Geometry check sheet. Reference: the model listing, model coordinates, mm. A direction names the side the tool comes from. Give positions to 0.01 mm unless a question says otherwise; leave off trailing zeros. Write each loop counter-clockwise with the first axis right and the second up, starting at its lowest first coordinate (ties: lowest second). Pieces come first, ordered by that corner, then holes. Notation, with made-up numbers: M 33,-9.5 L 64,-9.5 A10 cw 64,4.5 Z; hole C -6,-11 d8. An arc over 180 degrees is marked long. One line per item, written item: value. Start each with the question number.
1. Release check for a two-part mould opening along X. For faces 1 (the face through (4.62, 5.71, -1.97)), 2 (the face through (-6.2, 3, -2)), 3 (the face through (17, 3, -10)) record: pulls with the +X half, pulls with the -X half, needs draft (parallel to the pull), parting line crosses it, or undercut.
2. Cross-section at A-A on y = 4. Record the cut outline in (x, z).
3. Tool access check on faces 4 (the face through (4.5, 6.2, -3.6)), 5 (the face through (33.8, 3, -5)), 6 (the face through (7, 6, -4.497)), 7 (the face through (-3, 3, -7)). Record the directions out of +Z, -Z, +X, -X, +Y, -Y that give a thin tool (end or side, any length) a straight path to the whole face; none if there is none.
4. Cross-section at B-B on z = -5. Record the cut outline in (x, y), then the cut area to 3 significant figures.
5. Gauge pin test, flat ends, axial feed: pin 1 (3 mm diameter, centred on x = 37, y = 4.5, fed in from +Z); pin 2 (1 mm diameter, centred on y = 5, z = -4, fed in from +X). Record the tip position at first contact, or that the pin passes through.
6. Scan lines: line 1 (Z direction, x = 34.5, y = 1.75); line 2 (X direction, y = 2.5, z = -6.25). Record each from-to range of solid material in increasing order.
from build123d import *

# Parameters (mm, degrees)
BOSS_EXTRUDE1_DEPTH = 6.2
CUT_EXTRUDE1_DEPTH  = 1


with BuildPart() as part:
    # Sketch1 → Boss-Extrude1 (new body)
    with BuildSketch(Plane(origin=(0, 0, 0), x_dir=(1, 0, 0), z_dir=(0, 1, 0))):
        Polygon((0, 0), (33.7, 0), (39.9, 0), (39.9, 3), (33.8, 3), (33.8, 7), (39.9, 7), (39.9, 10), (33.7, 10), (0, 10), (-6.2, 10), (-6.2, 7), (0.1, 7), (0.1, 3), (-6.2, 3), (-6.2, 0), align=None)
    extrude(amount=BOSS_EXTRUDE1_DEPTH)

    # Sketch2 → Cut-Extrude1 (cut)
    with BuildSketch(Plane(origin=(0, 6.2, 0), x_dir=(1, 0, 0), z_dir=(0, 1, 0))):
        with BuildLine():
            Line((4.122268508, 1.240803577), (3.894574197, 1.399171966))
            Line((3.894574197, 1.399171966), (4.777366665, 2.689651734))
            add(Edge.make_bspline(
                [(4.777366665, 2.689651734), (4.721041498, 2.682763741), (4.610134103, 2.669200898), (4.498431161, 2.66670929), (4.443457411, 2.665483064)],
                knots=[0, 0, 0, 0, 0.000170115, 0.000334967, 0.000334967, 0.000334967, 0.000334967], degree=3))
            add(Edge.make_bspline(
                [(4.443457411, 2.665483064), (4.410127124, 2.666336755), (4.344702687, 2.668012475), (4.248516831, 2.681294687), (4.156092072, 2.701750875), (4.067673442, 2.732275102), (3.982928606, 2.770210192), (3.902042566, 2.817251911), (3.825124208, 2.872593333), (3.752999629, 2.935941833), (3.687402552, 3.00549978), (3.628961417, 3.079119542), (3.580391962, 3.157656315), (3.540045345, 3.239508014), (3.509447005, 3.325851097), (3.487165275, 3.415703053), (3.473447139, 3.509693614), (3.471815102, 3.573669982), (3.470986457, 3.606153136)],
                knots=[0, 0, 0, 0, 9.9954e-05, 0.000196201, 0.000290782, 0.000383503, 0.000476303, 0.000568919, 0.000663705, 0.000760153, 0.000856434, 0.000950205, 0.001041624, 0.001132931, 0.001223461, 0.001315861, 0.001410305, 0.001507717, 0.001507717, 0.001507717, 0.001507717], degree=3))
            add(Edge.make_bspline(
                [(3.470986457, 3.606153136), (3.472559837, 3.6505747), (3.475648063, 3.737765218), (3.500502432, 3.865158708), (3.541378597, 3.985615073), (3.598372911, 4.098817606), (3.670159408, 4.203137891), (3.756436486, 4.2971257), (3.856679368, 4.379444246), (3.968604485, 4.450205088), (4.089574726, 4.507114693), (4.216274151, 4.549060344), (4.34773196, 4.573733494), (4.436784061, 4.576986382), (4.481618468, 4.57862409)],
                knots=[0, 0, 0, 0, 0.000133185, 0.000261414, 0.000387724, 0.00051373, 0.000640399, 0.00076644, 0.000895188, 0.001028407, 0.001162697, 0.001295241, 0.001427846, 0.0015623, 0.0015623, 0.0015623, 0.0015623], degree=3))
            add(Edge.make_bspline(
                [(4.481618468, 4.57862409), (4.525604392, 4.57696387), (4.612516431, 4.573683434), (4.740322887, 4.54965869), (4.862733666, 4.509166851), (4.97907019, 4.45321014), (5.0867838, 4.383069031), (5.183644714, 4.299489856), (5.267442525, 4.202420556), (5.338039902, 4.094208854), (5.394709153, 3.977943093), (5.435596152, 3.856581963), (5.460765411, 3.730998266), (5.463937079, 3.645913279), (5.465537739, 3.602973048)],
                knots=[0, 0, 0, 0, 0.000131915, 0.000260652, 0.000388569, 0.000517718, 0.000646848, 0.000773094, 0.000900237, 0.001030248, 0.001159674, 0.001287189, 0.001413545, 0.001542287, 0.001542287, 0.001542287, 0.001542287], degree=3))
            add(Edge.make_bspline(
                [(5.465537739, 3.602973048), (5.464468754, 3.569641202), (5.462300585, 3.50203589), (5.447118363, 3.399319794), (5.421337195, 3.294589035), (5.392080297, 3.205941588), (5.363838974, 3.132727494), (5.337258661, 3.074895704), (5.307765493, 3.014025272), (5.273367756, 2.950754473), (5.23639053, 2.884276745), (5.194608186, 2.815258852), (5.148973846, 2.74360818), (5.116471172, 2.695305464), (5.099827603, 2.670571205)],
                knots=[0, 0, 0, 0, 9.9984e-05, 0.000202793, 0.000310776, 0.000423207, 0.000482616, 0.000546097, 0.000614079, 0.0006855, 0.000762103, 0.000842274, 0.000927493, 0.001016928, 0.001016928, 0.001016928, 0.001016928], degree=3))
            Line((5.099827603, 2.670571205), (4.122268508, 1.240803577))
        make_face()
        with BuildLine():
            add(Edge.make_bspline(
                [(4.496246874, 2.99112409), (4.521496301, 2.991813867), (4.570648352, 2.993156627), (4.642654901, 3.001329297), (4.710621857, 3.015819984), (4.774730776, 3.036611437), (4.835624466, 3.061699987), (4.892335707, 3.093642288), (4.944911961, 3.131757379), (4.993705294, 3.174583607), (5.037034066, 3.222163779), (5.075626672, 3.271963298), (5.108429472, 3.324200765), (5.134340445, 3.379530367), (5.15564431, 3.436605264), (5.170356364, 3.496344572), (5.178506438, 3.558437049), (5.179895795, 3.600617975), (5.180601842, 3.622053577)],
                knots=[0, 0, 0, 0, 7.5753e-05, 0.000147465, 0.000217073, 0.000283852, 0.000349411, 0.000414338, 0.000478589, 0.000543925, 0.000608743, 0.000671332, 0.000732749, 0.000793345, 0.000854313, 0.000915245, 0.00097749, 0.001041807, 0.001041807, 0.001041807, 0.001041807], degree=3))
            add(Edge.make_bspline(
                [(5.180601842, 3.622053577), (5.179994356, 3.64349813), (5.178797231, 3.685757253), (5.169193038, 3.74794166), (5.1522973, 3.807534833), (5.12962736, 3.864863023), (5.099764001, 3.919455217), (5.063928697, 3.971996815), (5.02135426, 4.022154674), (4.972366218, 4.068749145), (4.919539159, 4.111700453), (4.86324142, 4.149606394), (4.803937031, 4.181375622), (4.741987801, 4.207591116), (4.677264656, 4.228048798), (4.609805896, 4.242760265), (4.539270635, 4.250898928), (4.491390468, 4.252279503), (4.466990063, 4.252983064)],
                knots=[0, 0, 0, 0, 6.4316e-05, 0.000126743, 0.000188161, 0.000249812, 0.000311283, 0.000374438, 0.00044032, 0.000508243, 0.00057698, 0.000644365, 0.000711521, 0.0007785, 0.000845884, 0.000914871, 0.00098532, 0.001058531, 0.001058531, 0.001058531, 0.001058531], degree=3))
            add(Edge.make_bspline(
                [(4.466990063, 4.252983064), (4.442801867, 4.252278367), (4.395344825, 4.250895757), (4.325436623, 4.242775735), (4.258433992, 4.22794986), (4.193898379, 4.207600592), (4.13195099, 4.181373666), (4.072649399, 4.149604729), (4.016338491, 4.111709179), (3.96356208, 4.06871535), (3.914487536, 4.022371556), (3.872645092, 3.971777089), (3.836727776, 3.919482549), (3.806905452, 3.864855759), (3.784224597, 3.807536771), (3.767331781, 3.747941135), (3.757726803, 3.68575739), (3.756529786, 3.643498177), (3.755922355, 3.622053577)],
                knots=[0, 0, 0, 0, 7.2576e-05, 0.000142393, 0.000210758, 0.000278143, 0.000345121, 0.000412278, 0.000479663, 0.0005484, 0.000616323, 0.000681795, 0.00074495, 0.000806421, 0.000868072, 0.00092949, 0.000991917, 0.001056233, 0.001056233, 0.001056233, 0.001056233], degree=3))
            add(Edge.make_bspline(
                [(3.755922355, 3.622053577), (3.756472016, 3.600601282), (3.757556049, 3.558293431), (3.768013401, 3.496130203), (3.785501555, 3.436541627), (3.808923431, 3.3789483), (3.839767731, 3.323910258), (3.877617221, 3.271688436), (3.921981538, 3.221690849), (3.97226763, 3.174694307), (4.027302319, 3.131557691), (4.086082225, 3.093883702), (4.147595434, 3.062067984), (4.212058485, 3.036539729), (4.278993653, 3.01602772), (4.349002522, 3.001356004), (4.421853566, 2.993235019), (4.471211193, 2.991834484), (4.496246874, 2.99112409)],
                knots=[0, 0, 0, 0, 6.4316e-05, 0.000126844, 0.000188436, 0.000250326, 0.000312966, 0.000377217, 0.000443451, 0.000513196, 0.000583426, 0.000652939, 0.000722346, 0.000790847, 0.000860662, 0.000932137, 0.001005113, 0.00108023, 0.00108023, 0.00108023, 0.00108023], degree=3))
        make_face(mode=Mode.SUBTRACT)
        Polygon((6.076114662, 4.497213833), (8.029960816, 4.497213833), (6.36105056, 1.240803577), (6.114911738, 1.376275332), (7.547859454, 4.171572808), (6.076114662, 4.171572808), align=None)
    extrude(amount=-CUT_EXTRUDE1_DEPTH, mode=Mode.SUBTRACT)


solid = part.part
Report:
1. face 1: undercut
1. face 2: pulls with the -X half
1. face 3: needs draft
2. outline: M -6.2,-10 L 39.9,-10 L 39.9,-7 L 33.8,-7 L 33.8,-3 L 39.9,-3 L 39.9,0 L -6.2,0 L -6.2,-3 L 0.1,-3 L 0.1,-7 L -6.2,-7 Z
3. face 4: +Z, -Z, +X, -X, +Y
3. face 5: +X, +Y, -Y
3. face 6: +Y
3. face 7: -X, +Y, -Y
4. outline: M 0.1,0 L 33.8,0 L 33.8,6.2 L 0.1,6.2 Z
4. area: 209 mm^2
5. pin 1: stops at z = 0
5. pin 2: stops at x = 33.8
6. line 1: z = -10 to -7, -3 to 0
6. line 2: x = 0.1 to 33.8
